The drawing under review shows one solid part. Ordinate dimensions are in mm from its lowest x, y, z. A direction names the side the tool comes from. Give positions to 0.01 mm unless a question says otherwise; leave off trailing zeros. Order: outer loops, then holes, each group sorted by start corner. A loop starts at its lowest first (then second) coordinate and runs counter-clockwise, first axis right, second up. Notation, with made-up numbers: (3.5, 48.5) - (30.5, 48.5) arc R18 ccw to (30.5, 52.5) - close; hole circle Ø4 at (4, -27). An arc over 180 degrees is marked (long way). Use CSV: the item, a comma, the result in double quotes.
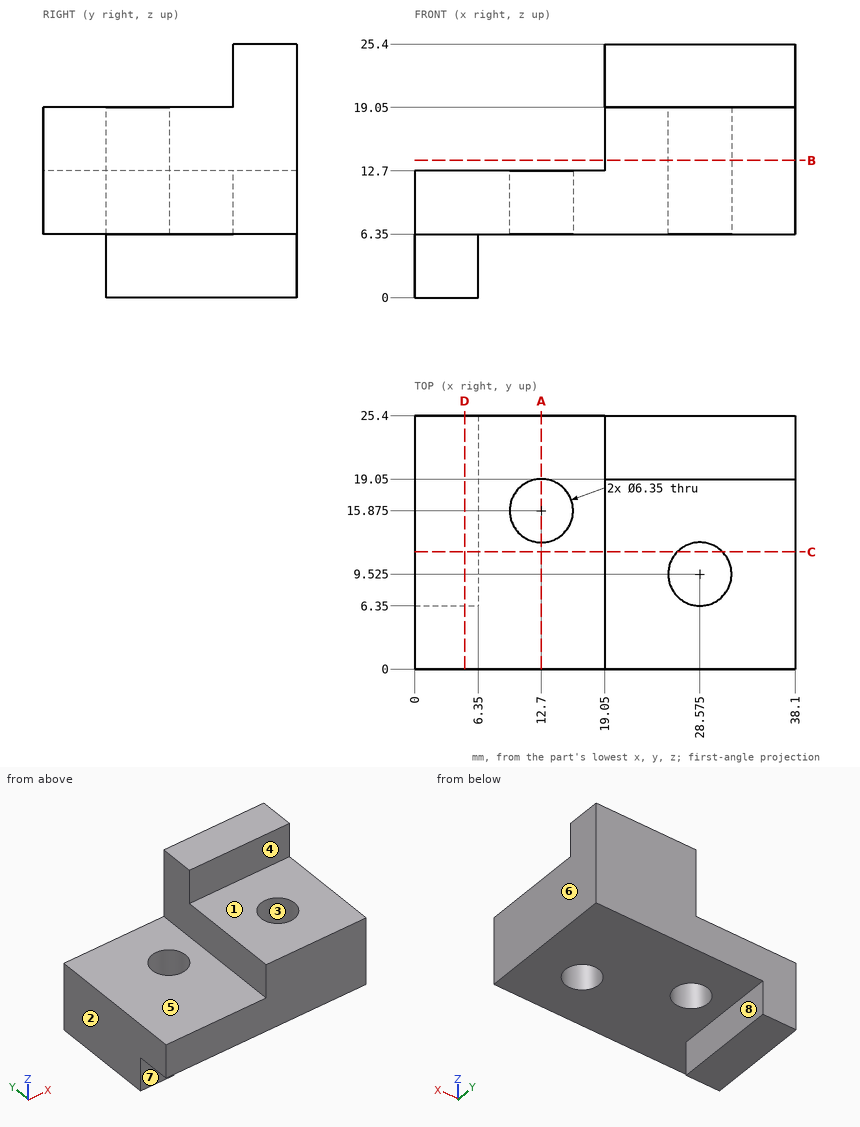
Item 1: Wall thickness on L1, parallel to Y at x = 12.7, z = 9.25; L2, parallel to Z at x = 3, y = 22.75; L3, parallel to X at y = 16.75, z = 14.5: over which ranges is each line inside the solid? List them lowest first.
Results list:
L1,"y = 0 to 12.7, 19.05 to 25.4"
L2,"z = 0 to 12.7"
L3,"x = 19.05 to 38.1"
Item 2: Mouldability with a two-part tool opening along X and no side actions: class the marked faces 1, 2 and 3 as pulls with the +X half, pulls with the -X half, needs draft (parallel to the pull), parting line crosses it, or undercut.
Results list:
face 1,"needs draft"
face 2,"pulls with the -X half"
face 3,"undercut"
Item 3: Take a section at D-D, the plane x = 5. Give the boundary of the cut face in (y, z).
Results list:
outline,"(0, 6.35) - (6.35, 6.35) - (6.35, 0) - (25.4, 0) - (25.4, 12.7) - (0, 12.7) - close"
Item 4: Tool access review of the marked faces 4, 5, 6, 7 and 8: name each direction out of +Z, -Z, +X, -X, +Y, -Y from which nothing blocks a thin tool from reaching the whole face with its end or side.
Results list:
face 4,"+Z, +X, -X, -Y"
face 5,"+Z, -X, +Y, -Y"
face 6,"+Z, -Z, +X, +Y, -Y"
face 7,"-Z, +X, -X, -Y"
face 8,"-Z, +X, +Y, -Y"
Item 5: Take a section at C-C, the plane y = 11.75. Give the boundary of the cut face in (x, z), and give its area (3 significant figures).
Results list:
outline,"(0, 0) - (6.35, 0) - (6.35, 6.35) - (26.31, 6.35) - (26.31, 19.05) - (19.05, 19.05) - (19.05, 12.7) - (0, 12.7) - close; (30.84, 6.35) - (38.1, 6.35) - (38.1, 19.05) - (30.84, 19.05) - close"
area,"346 mm2"
Item 6: Take a section at B-B, the plane z = 13.75. Give the boundary of the cut face in (x, y) (3 decimals), and give its area (3 significant figures).
Results list:
outline,"(19.05, 0) - (38.1, 0) - (38.1, 25.4) - (19.05, 25.4) - close; hole circle Ø6.35 at (28.575, 9.525)"
area,"452 mm2"
Item 7: Clearance check with flat-ended pins moving along their axes: pin 1 (7.5 mm diameter, centred on x = 12.7, y = 15.875, fed in from +Z); pin 2 (7.5 mm diameter, centred on x = 15.5, y = 8.5, fed in from -Z); pin 3 (5 mm diameter, centred on x = 3.5, z = 4.5, fed in from -Y); pin 4 (9.5 mm diameter, centred on x = 31.5, y = 11.5, fed in from +Z). State where each tip first meets the part, or that it passes through.
Results list:
pin 1,"stops at z = 12.7"
pin 2,"stops at z = 6.35"
pin 3,"stops at y = 0"
pin 4,"stops at z = 19.05"
Item 8: Take a section at A-A, the plane x = 12.7. Give the boundary of the cut face in (y, z), and give its area (3 significant figures).
Results list:
outline,"(0, 6.35) - (12.7, 6.35) - (12.7, 12.7) - (0, 12.7) - close; (19.05, 6.35) - (25.4, 6.35) - (25.4, 12.7) - (19.05, 12.7) - close"
area,"121 mm2"
